```python
from build123d import *

# Parameters (mm, degrees)
EXTRUDE_1_DEPTH = 2.2
FILLET_1_R      = 1


with BuildPart() as part:
    # 草图1 → 凸台-拉伸1 (new body)
    with BuildSketch(Plane(origin=(0, 0, 0), x_dir=(1, 0, 0), z_dir=(0, 1, 0))):
        Polygon((18.75, 4.15), (-18.75, 4.15), (-18.75, -9.15), (-12.75, -9.15), (-8.75, -5.15), (8.75, -5.15), (12.75, -9.15), (18.75, -9.15), align=None)
        with BuildLine():
            Line((-13.45, -6.15), (-15.75, -6.15))
            ThreePointArc((-15.75, -6.15), (-16.755, -5.145), (-15.75, -4.14))
            Line((-15.75, -4.14), (-15.75, -1.96))
            ThreePointArc((-15.75, -1.96), (-16.755, -0.955), (-15.75, 0.05))
            Line((-15.75, 0.05), (-13.45, 0.05))
            ThreePointArc((-13.45, 0.05), (-12.739357685, -0.244357685), (-12.445, -0.955))
            ThreePointArc((-12.445, -0.955), (-12.739357685, -1.665642315), (-13.45, -1.96))
            Line((-13.45, -1.96), (-13.45, -4.14))
            ThreePointArc((-13.45, -4.14), (-12.739357685, -4.434357685), (-12.445, -5.145))
            ThreePointArc((-12.445, -5.145), (-12.739357685, -5.855642315), (-13.45, -6.15))
        make_face(mode=Mode.SUBTRACT)
        with BuildLine():
            Line((13.45, 0.05), (15.75, 0.05))
            ThreePointArc((15.75, 0.05), (16.460642315, -0.244357685), (16.755, -0.955))
            ThreePointArc((16.755, -0.955), (16.460642315, -1.665642315), (15.75, -1.96))
            Line((15.75, -1.96), (15.75, -4.14))
            ThreePointArc((15.75, -4.14), (16.460642315, -4.434357685), (16.755, -5.145))
            ThreePointArc((16.755, -5.145), (16.460642315, -5.855642315), (15.75, -6.15))
            Line((15.75, -6.15), (13.45, -6.15))
            ThreePointArc((13.45, -6.15), (12.445, -5.145), (13.45, -4.14))
            Line((13.45, -4.14), (13.45, -1.96))
            ThreePointArc((13.45, -1.96), (12.445, -0.955), (13.45, 0.05))
        make_face(mode=Mode.SUBTRACT)
        with BuildLine():
            Line((5.09, -1.15), (-5.09, -1.15))
            ThreePointArc((-5.09, -1.15), (-6.095, -2.155), (-7.1, -1.15))
            Line((-7.1, -1.15), (-7.1, 1.15))
            ThreePointArc((-7.1, 1.15), (-6.095, 2.155), (-5.09, 1.15))
            Line((-5.09, 1.15), (5.09, 1.15))
            ThreePointArc((5.09, 1.15), (6.095, 2.155), (7.1, 1.15))
            Line((7.1, 1.15), (7.1, -1.15))
            ThreePointArc((7.1, -1.15), (6.095, -2.155), (5.09, -1.15))
        make_face(mode=Mode.SUBTRACT)
    extrude(amount=EXTRUDE_1_DEPTH)

    # 圆角1
    fillet_1_edges = [part.edges().sort_by_distance(p)[0] for p in [
        (-18.75, 1.1, 9.15),
        (-18.75, 1.1, -4.15),
        (18.75, 1.1, -4.15),
        (18.75, 1.1, 9.15),
        (12.75, 1.1, 9.15),
        (8.75, 1.1, 5.15),
        (-8.75, 1.1, 5.15),
        (-12.75, 1.1, 9.15),
    ]]
    fillet(fillet_1_edges, radius=FILLET_1_R)


solid = part.part
```
CAD build for the part. Positions are in the model's coordinates, mm. A direction names the side the tool comes from. Round coordinates to 2 decimals unless told otherwise and drop trailing zeros. Order: outer loops, then holes, each group sorted by start corner. A loop starts at its lowest first (then second) coordinate and runs counter-clockwise, first axis right, second up.
Item 1: Saw through at D-D on y = 1.7. State how many separate pieces and enclosed holes the cut face has, then the cut area to 3 significant figures.
Item 2: Mould opens along X. For faces 4 (the face through (-15.75, 1, 3)), 5 (the face through (0, 1, -4.15)), 6 (the face through (18.75, 1, 3)) say: pulls with the +X half, pulls with the -X half, needs draft (parallel to the pull), parting line crosses it, or undercut.
Item 3: Saw through at A-A on z = 3. Write the cut outline in (x, y).
Item 4: Saw through at C-C on z = 7.25. Write the cut outline in (x, y).
Item 5: Saw through at B-B on x = -0.5. Write the cut outline in (y, z), then the cut area to 3 significant figures.
Item 6: Probe line 1 along X through (y, z) = (1.35, 3); line 2 along Z through (x, y) = (-6, 0.6); line 3 along Z through (x, y) = (2, 1.45). List the from-to ranges inside material, lowest first.
Item 7: Pin check, flat tips, straight feed: pin 1 (1.1 mm diameter, centred on x = 1.5, y = 1.5, fed in from +Z); pin 2 (1.1 mm diameter, centred on x = -1.5, y = 1.5, fed in from +Z). Stop position of each tip, or through.
Item 8: Tool access for faces 1 (the face through (7.1, 1, 0)), 2 (the face through (15, 1, 9.15)), 3 (the face through (0, 1, 5.15)): list every direction of +Z, -Z, +X, -X, +Y, -Y with a clear straight run to the whole face (end or side of a thin tool).
Reported:
1. separate pieces: 1
1. enclosed holes: 3
1. area: 332 mm2
2. face 4: undercut
2. face 5: needs draft
2. face 6: pulls with the +X half
3. outline: (-18.75, 0) - (-15.75, 0) - (-15.75, 2.2) - (-18.75, 2.2) - close; (-13.45, 0) - (13.45, 0) - (13.45, 2.2) - (-13.45, 2.2) - close; (15.75, 0) - (18.75, 0) - (18.75, 2.2) - (15.75, 2.2) - close
4. outline: (-18.75, 0) - (-10.85, 0) - (-10.85, 2.2) - (-18.75, 2.2) - close; (10.85, 0) - (18.75, 0) - (18.75, 2.2) - (10.85, 2.2) - close
5. outline: (0, -4.15) - (2.2, -4.15) - (2.2, -1.15) - (0, -1.15) - close; (0, 1.15) - (2.2, 1.15) - (2.2, 5.15) - (0, 5.15) - close
5. area: 15.4 mm2
6. line 1: x = -18.75 to -15.75, -13.45 to 13.45, 15.75 to 18.75
6. line 2: z = -4.15 to -2.15, 2.15 to 5.15
6. line 3: z = -4.15 to -1.15, 1.15 to 5.15
7. pin 1: stops at z = 5.15
7. pin 2: stops at z = 5.15
8. face 1: +Y, -Y
8. face 2: +Z, +X, -X, +Y, -Y
8. face 3: +Z, +Y, -Y
